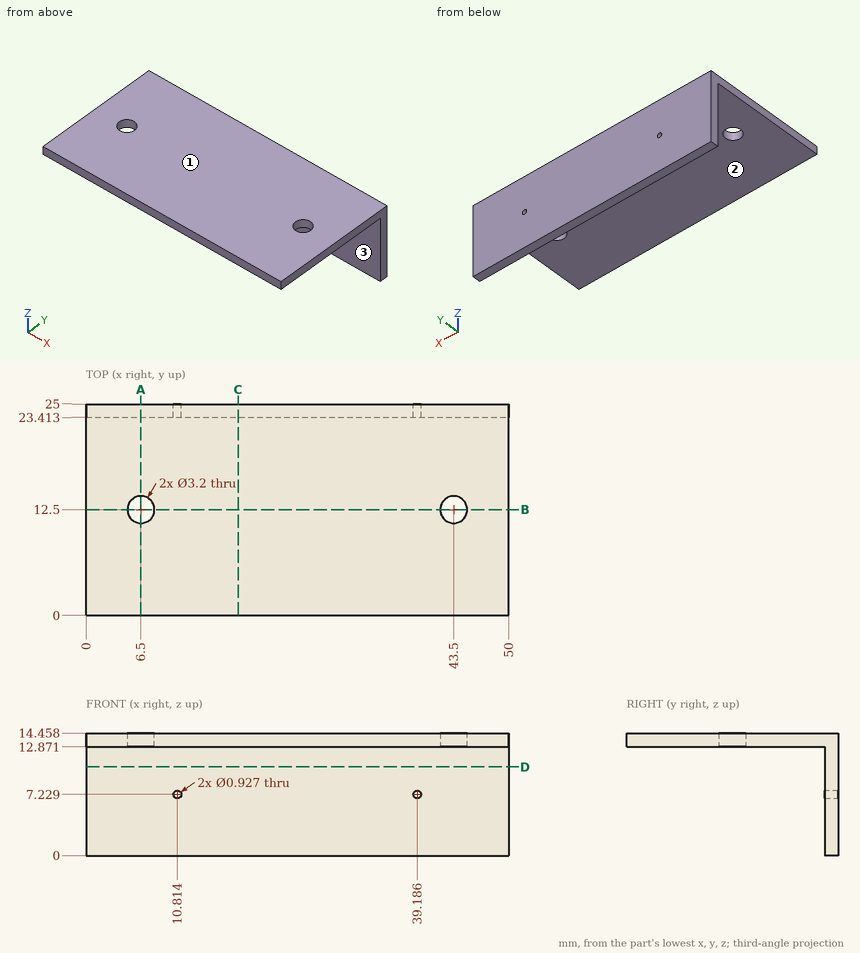
For this review, use the dimensioned drawing (mm, ordinates from the lowest corner) and the shaded views. Coordinates: 2 decimals unless noted, no trailing zeros. Loops run counter-clockwise (first coordinate to the right, second up) from the corner with the lowest first, then second, coordinate; pieces in that order, holes last. Notation, with made-up numbers: (23.5, 34) -> (55.5, 34) arc R17 cw to (55.5, 41) -> close; hole circle Ø7 at (-15, -11.5). An arc over 180 degrees is marked (long way). Use a Markdown table: item, result. Add a question column.
Item 1: We need section A-A, the plane x = 6.5. Write out the cut boundary in (y, z).
Item 2: We need section D-D, the plane z = 10.5. Write out the cut boundary in (x, y).
Item 3: The part is to be moulded in two halves that separate along Z. For the marked faces 1, 2 and 3, say which applies: +Z half, -Z half, draft (parallel to the pull), parting line (faces both ways), or undercut.
Item 4: Clearance check with flat-ended pins moving along their axes: P1, Ø1, axis at x = 13.5, z = 8, coming from the -Y side; P2, Ø1.5, axis at y = 8, z = 10.5, coming from the +X side; P3, Ø3, axis at x = 20, y = 10, coming from the -Z side. State where each tip first meets the part, or that it passes through.
Item 5: We need section C-C, the plane x = 18. Write out the cut boundary in (y, z).
Item 6: Wall thickness on L1, parallel to Y at x = 6.5, z = 13.7; L2, parallel to Z at x = 22, y = 11.75; L3, parallel to Y at x = 38.5, z = 9.25: over which ranges is each line inside the solid? List them lowest first. Write a range as from..to.
Item 7: We need section B-B, the plane y = 12.5. Write out the cut boundary in (x, z).
Numbers:
| question | item | result |
|---|---|---|
| 1 | outline | (0, 12.87) -> (10.9, 12.87) -> (10.9, 14.46) -> (0, 14.46) -> close; (14.1, 12.87) -> (23.41, 12.87) -> (23.41, 0) -> (25, 0) -> (25, 14.46) -> (14.1, 14.46) -> close |
| 2 | outline | (0, 23.41) -> (50, 23.41) -> (50, 25) -> (0, 25) -> close |
| 3 | face 1 | +Z half |
| 3 | face 2 | -Z half |
| 3 | face 3 | draft |
| 4 | P1 | stops at y = 23.41 |
| 4 | P2 | passes through |
| 4 | P3 | stops at z = 12.87 |
| 5 | outline | (0, 12.87) -> (23.41, 12.87) -> (23.41, 0) -> (25, 0) -> (25, 14.46) -> (0, 14.46) -> close |
| 6 | L1 | y = 0..10.9, 14.1..25 |
| 6 | L2 | z = 12.87..14.46 |
| 6 | L3 | y = 23.41..25 |
| 7 | outline | (0, 12.87) -> (4.9, 12.87) -> (4.9, 14.46) -> (0, 14.46) -> close; (8.1, 12.87) -> (41.9, 12.87) -> (41.9, 14.46) -> (8.1, 14.46) -> close; (45.1, 12.87) -> (50, 12.87) -> (50, 14.46) -> (45.1, 14.46) -> close |
